Could you check a few things on this model? Use its own coordinates, in mm. A direction names the side the tool comes from. Coordinates: 2 decimals unless noted, no trailing zeros. Order: outer loops, then holes, each group sorted by start corner. A loop starts at its lowest first (then second) coordinate and runs counter-clockwise, first axis right, second up. Notation, with made-up numbers: M 70,-33.5 L 93,-33.5 A9 ccw 93,-26.5 Z; hole C -23.5,-2.75 d2. An arc over 180 degrees is marked long. Put each result on its own line as item: value. Start each with the question number.
```python
from build123d import *

# Parameters (mm, degrees)
BOSS_EXTRUDE1_DEPTH     = 12
BOSS_EXTRUDE2_DEPTH     = 2
BOSS_EXTRUDE3_DEPTH     = 2
SKETCH3_R               = 1.5875
CUT_EXTRUDE1_DEPTH      = 12
CUT_EXTRUDE1_DEPTH_BACK = 2
FILLET1_R               = 0.5


with BuildPart() as part:
    # Sketch1 → Boss-Extrude1 (new body)
    with BuildSketch(Plane(origin=(0, 0, 0), x_dir=(1, 0, 0), z_dir=(0, 1, 0))):
        Polygon((15, 0), (0, 0), (0, 15), (2, 15), (2, 2), (15, 2), align=None)
    extrude(amount=BOSS_EXTRUDE1_DEPTH)

    # Sketch1_3 → Boss-Extrude2 (add)
    with BuildSketch(Plane(origin=(0, 0, 0), x_dir=(1, 0, 0), z_dir=(0, 1, 0))):
        with BuildLine():
            Line((0, 15), (-3, 15))
            ThreePointArc((-3, 15), (-5.121320344, 14.121320344), (-6, 12))
            Line((-6, 12), (-6, -1))
            ThreePointArc((-6, -1), (-4.535533906, -4.535533906), (-1, -6))
            Line((-1, -6), (12, -6))
            ThreePointArc((12, -6), (14.121320344, -5.121320344), (15, -3))
            Line((15, -3), (15, 0))
            Line((15, 0), (0, 0))
            Line((0, 0), (0, 15))
        make_face()
    extrude(amount=BOSS_EXTRUDE2_DEPTH)

    # Sketch2 → Boss-Extrude3 (add)
    with BuildSketch(Plane(origin=(0, 12, 0), x_dir=(1, 0, 0), z_dir=(0, 1, 0))):
        Polygon((2, 15), (15, 2), (15, 0), (0, 0), (0, 15), align=None)
    extrude(amount=BOSS_EXTRUDE3_DEPTH)

    # Sketch3 → Cut-Extrude1 (cut, two sides)
    with BuildSketch(Plane(origin=(0, 0, 0), x_dir=(1, 0, 0), z_dir=(0, 1, 0))) as cut_extrude1_sk:
        with Locations((-2.5, -2.5)):
            Circle(SKETCH3_R)
        with Locations((-2.5, 11.5)):
            Circle(SKETCH3_R)
        with Locations((11.5, -2.5)):
            Circle(SKETCH3_R)
    extrude(amount=CUT_EXTRUDE1_DEPTH, mode=Mode.SUBTRACT)
    extrude(cut_extrude1_sk.sketch, amount=-CUT_EXTRUDE1_DEPTH_BACK, mode=Mode.SUBTRACT)

    # Fillet1
    fillet1_edges = [part.edges().sort_by_distance(p)[0] for p in [
        (0, 8, 0),
        (7.5, 2, 0),
        (0, 2, -7.5),
        (0, 14, -7.5),
        (7.5, 14, 0),
    ]]
    fillet(fillet1_edges, radius=FILLET1_R)


solid = part.part
```
Item 1: For pin 1 Ø3.5 at (x, z) = (11.5, 2.5) entering from -Y; pin 2 Ø6.5 at (x, z) = (6.5, -11.5) entering from -Y; pin 3 Ø5 at (x, z) = (-2.5, 2.5) entering from +Y; pin 4 Ø1 at (x, y) = (4.5, 11) entering from -Z, each with a flat end and sliding along its axis, tell me the tip position at first contact or that it passes through.
Item 2: If we section it at C-C on z = -6.5: Write out the boundary of the cut face in (x, y), then the cut area to 3 significant figures.
Item 3: If we section it at D-D on y = 11: Write out the boundary of the cut face in (x, z).
Item 4: For faces 4 (the flat face through (8, 8, 0)), 5 (the flat face through (1, 2, 1)), 6 (the flat face through (0, 8, -8)), 7 (the flat face through (1, 7, -15)), 8 (the flat face through (8, 6, -2)), which set-ups out of +Z, -Z, +X, -X, +Y, -Y let a thin tool reach every point of the face, with its end or its side?
Item 5: If we mould it in two halves opening along X, with no side actions, what happens to faces 1 (the cylindrical face through (9.914, 0.986, 2.43)), 2 (the flat face through (6, 12, -6)), 3 (the cylindrical face through (14.1, 0.99, 5.14))? For each: released by +X, released by -X, zero draft, split by the parting line, or undercut.
Item 6: If we section it at A-A on x = 11.5: Write out the boundary of the cut face in (y, z).
Item 7: I need wall thicknesses on probe 1 along Z at (x, y) = (-2.5, 0.7); probe 2 along Z at (x, y) = (-3, 1.5); probe 3 along Z at (x, y) = (11.5, 1.35). Which ranges of each line are inside material? Lowest first, please.
Item 8: If we section it at B-B on z = -11.5: Write out the boundary of the cut face in (x, y), then the cut area to 4 significant figures.
Geometry check:
1. pin 1: stops at y = 0
1. pin 2: stops at y = 12
1. pin 3: stops at y = 2
1. pin 4: stops at z = -2
2. outline: M -6,0 L 2,0 L 2,12 L 10.5,12 L 10.5,14 L 0.5,14 A0.5 ccw 0,13.5 L 0,2.5 A0.5 cw -0.5,2 L -6,2 Z
2. area: 57.0 mm²
3. outline: M 0,-15 L 2,-15 L 2,-2 L 15,-2 L 15,0 L 0.5,0 A0.5 ccw 0,-0.5 Z
4. face 4: +Z, +X, -X, +Y
4. face 5: +Z, -X, +Y
4. face 6: +Z, -Z, -X, +Y
4. face 7: -Z, +X, -X, +Y, -Y
4. face 8: -Z, +X, -Y
5. face 1: undercut
5. face 2: zero draft
5. face 3: released by +X
6. outline: M 0,-2 L 12,-2 L 12,-5.5 L 14,-5.5 L 14,-0.5 A0.5 ccw 13.5,0 L 2.5,0 A0.5 cw 2,0.5 L 2,0.91 L 0,0.91 Z; M 0,4.09 L 2,4.09 L 2,6 L 0,6 Z
7. probe 1: z = -15 to -13.09, -9.91 to 0.91, 4.09 to 5.77
7. probe 2: z = -15 to -13.01, -9.99 to 0.99, 4.01 to 5.58
7. probe 3: z = -2 to 0.91, 4.09 to 6
8. outline: M -6,0 L -4.09,0 L -4.09,2 L -6,2 Z; M -0.91,0 L 2,0 L 2,12 L 5.5,12 L 5.5,14 L 0.5,14 A0.5 ccw 0,13.5 L 0,2.5 A0.5 cw -0.5,2 L -0.91,2 Z
8. area: 40.65 mm²
